Work out the finished part from the listing and answer in its coordinate system (mm). Face numbers are marked on the shaded views. Coordinates: 2 decimals unless noted, no trailing zeros. Order: outer loops, then holes, each group sorted by start corner. A loop starts at its lowest first (then second) coordinate and runs counter-clockwise, first axis right, second up. Notation, with made-up numbers: M 59,-4.75 L 63,-4.75 A11 ccw 63,6.25 Z; hole C 1,-23 d11. An arc over 180 degrees is marked long. Use a Markdown table: item, result.
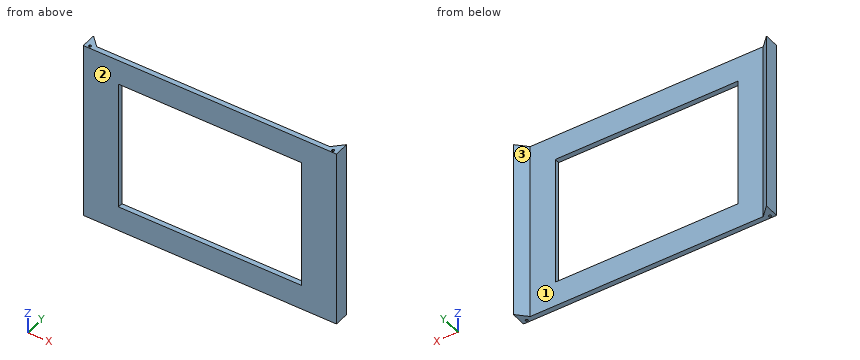
from build123d import *

# Parameters (mm, degrees)
BOSS_EXTRUDE1_DEPTH      = 90
BOSS_EXTRUDE1_DEPTH_BACK = 90
CUT_EXTRUDE1_DEPTH       = 221.229425827
SKETCH5_W                = 182
SKETCH5_H                = 130
CUT_EXTRUDE3_DEPTH       = 156.164428913


with BuildPart() as part:
    # Sketch1 → Boss-Extrude1 (new, two sides: drawn at the far end of the back side and taken through both)
    with BuildSketch(Plane.XY.offset(-BOSS_EXTRUDE1_DEPTH_BACK)):
        Polygon((-126, 0), (126, 0), (126, 15), (116, 5), (-116, 5), (-126, 15), align=None)
    extrude(amount=BOSS_EXTRUDE1_DEPTH + BOSS_EXTRUDE1_DEPTH_BACK)

    # Sketch3 → Cut-Extrude1 (cut, through all)
    with BuildSketch(Plane.XY.offset(90)):
        Polygon((-121, 3.943375673), (-122.25, 3.221687836), (-122.25, 1.778312164), (-121, 1.056624327), (-119.75, 1.778312164), (-119.75, 3.221687836), align=None)
        Polygon((119.75, 3.221687836), (121, 3.943375673), (122.25, 3.221687836), (122.25, 1.778312164), (121, 1.056624327), (119.75, 1.778312164), align=None)
    extrude(amount=-CUT_EXTRUDE1_DEPTH, mode=Mode.SUBTRACT)

    # Sketch5 → Cut-Extrude3 (cut, through all)
    with BuildSketch(Plane(origin=(0, 5, 0), x_dir=(1, 0, 0), z_dir=(0, 1, 0))):
        Rectangle(SKETCH5_W, SKETCH5_H)
    extrude(amount=-CUT_EXTRUDE3_DEPTH, mode=Mode.SUBTRACT)


solid = part.part
1. Section B-B on y = 11.5 is taken. Determine the outline of the cut face in (x, z).
Answers below:
| item | result |
|---|---|
| outline | M -126,-90 L -122.5,-90 L -122.5,90 L -126,90 Z; M 122.5,-90 L 126,-90 L 126,90 L 122.5,90 Z |
2. Section C-C on x = -82 is taken. Determine the outline of the cut face in (y, z), then the cut area to 3 significant figures.
Answers below:
| item | result |
|---|---|
| outline | M 0,-90 L 5,-90 L 5,-65 L 0,-65 Z; M 0,65 L 5,65 L 5,90 L 0,90 Z |
| area | 250 mm² |
3. A flat-ended cylindrical pin translates along its axis: P1, Ø12, axis at x = 80.5, z = -28, coming from the +Y side. Find the tip coordinate at first contact, or state that the pin passes through.
Answers below:
| item | result |
|---|---|
| P1 | through |
4. Find the intervals of material crossed by probe 1 along X at (y, z) = (2, 29); probe 2 along Z at (x, y) = (34, 0.5); probe 3 along X at (y, z) = (2.5, 79), in increasing order.
Answers below:
| item | result |
|---|---|
| probe 1 | -126 to -122.25, -119.75 to -91, 91 to 119.75, 122.25 to 126 |
| probe 2 | -90 to -65, 65 to 90 |
| probe 3 | -126 to -122.25, -119.75 to 119.75, 122.25 to 126 |
5. Section D-D on z = 67.5 is taken. Determine the outline of the cut face in (x, y).
Answers below:
| item | result |
|---|---|
| outline | M -126,0 L 126,0 L 126,15 L 116,5 L -116,5 L -126,15 Z; hole M -122.25,1.78 L -121,1.06 L -119.75,1.78 L -119.75,3.22 L -121,3.94 L -122.25,3.22 Z; hole M 119.75,1.78 L 121,1.06 L 122.25,1.78 L 122.25,3.22 L 121,3.94 L 119.75,3.22 Z |
6. For a pull along X with two mould halves and no side action, classify the marked faces 1, 2 and 3 as +X half, -X half, draft (parallel to the pull), parting line (faces both ways), or undercut.
Answers below:
| item | result |
|---|---|
| face 1 | undercut |
| face 2 | draft |
| face 3 | undercut |
7. Section A-A on z = -34.5 is taken. Determine the outline of the cut face in (x, y).
Answers below:
| item | result |
|---|---|
| outline | M -126,0 L -91,0 L -91,5 L -116,5 L -126,15 Z; M 91,0 L 126,0 L 126,15 L 116,5 L 91,5 Z; hole M -122.25,1.78 L -121,1.06 L -119.75,1.78 L -119.75,3.22 L -121,3.94 L -122.25,3.22 Z; hole M 119.75,1.78 L 121,1.06 L 122.25,1.78 L 122.25,3.22 L 121,3.94 L 119.75,3.22 Z |
